Model file for the job. Use its own axes, mm. A direction names the side the tool comes from. Give positions to 0.01 mm unless a question says otherwise; leave off trailing zeros. Write each loop counter-clockwise with the first axis right and the second up, starting at its lowest first coordinate (ties: lowest second). Pieces come first, ordered by that corner, then holes. Notation, with made-up numbers: (-23, 36) - (7, 36) arc R16 ccw to (7, 52) - close; hole circle Ø2 at (-9, 88.5). An arc over 180 degrees is marked (long way). Use CSV: the item, a comma, the result in double quotes.
from build123d import *

# Parameters (mm, degrees)
BOSS_EXTRUDE1_DEPTH         = 1.524
KES_EKSTR_ZYON1_DEPTH       = 2.54
RADYUS1_R                   = 0.508
Y_KSEKLIK_EKSTR_ZYON1_DEPTH = 6.223
Y_KSEKLIK_EKSTR_ZYON2_START = -1.524
Y_KSEKLIK_EKSTR_ZYON2_DEPTH = 1.524
IZIM5_W                     = 1.905
IZIM5_H                     = 23.876
KES_EKSTR_ZYON2_DEPTH       = 9.779
RADYUS2_R                   = 0.254


with BuildPart() as part:
    # Sketch2 → Boss-Extrude1 (new body)
    with BuildSketch(Plane(origin=(0, 0, 0), x_dir=(0, 0, -1), z_dir=(1, 0, 0))):
        with BuildLine():
            Line((-10.16, 10.851579944), (-10.16, 9.756379827))
            ThreePointArc((-10.16, 9.756379827), (-8.902698353, 7.16361824), (-6.088278228, 6.54534691))
            ThreePointArc((-6.088278228, 6.54534691), (-1.097578785, 7.201770952), (3.920718614, 6.808496661))
            ThreePointArc((3.920718614, 6.808496661), (7.044965017, 7.926917254), (7.619757818, 11.195157369))
            ThreePointArc((7.619757818, 11.195157369), (4.593793799, 26.843864795), (6.687175028, 42.644379261))
            ThreePointArc((6.687175028, 42.644379261), (5.465660141, 45.611386582), (2.312998216, 45.014767901))
            ThreePointArc((2.312998216, 45.014767901), (-6.944233805, 29.036045126), (-10.16, 10.851579944))
        make_face()
    extrude(amount=BOSS_EXTRUDE1_DEPTH)

    # Sketch3 → Kes-Ekstrüzyon1 (cut)
    with BuildSketch(Plane(origin=(1.524, 0, 0), x_dir=(0, 0, -1), z_dir=(1, 0, 0))):
        with BuildLine():
            Line((-7.62, 10.851579944), (-7.62, 9.756379827))
            ThreePointArc((-7.62, 9.756379827), (-7.329853466, 9.15805023), (-6.680371899, 9.015372231))
            ThreePointArc((-6.680371899, 9.015372231), (-1.164335672, 9.74089354), (4.382203558, 9.306221955))
            ThreePointArc((4.382203558, 9.306221955), (5.103183497, 9.564319015), (5.23582799, 10.318528273))
            ThreePointArc((5.23582799, 10.318528273), (2.05490982, 26.768577734), (4.25548932, 43.378207999))
            ThreePointArc((4.25548932, 43.378207999), (-4.558282485, 28.164933022), (-7.62, 10.851579944))
        make_face()
    extrude(amount=-KES_EKSTR_ZYON1_DEPTH, mode=Mode.SUBTRACT)

    # Radyus1
    radyus1_edges = [part.edges().sort_by_distance(p)[0] for p in [
        (0.762, 43.378207999, -4.25548932),
    ]]
    fillet(radyus1_edges, radius=RADYUS1_R)

    # Çizim3 → Yükseklik-Ekstrüzyon1 (add)
    with BuildSketch(Plane.ZY):
        with BuildLine():
            Line((8.89, 9.756379827), (8.89, 10.851579944))
            ThreePointArc((8.89, 10.851579944), (6.172491894, 27.401227257), (-1.694641367, 42.212840631))
            ThreePointArc((-1.694641367, 42.212840631), (-3.87996363, 42.737551733), (-4.833471032, 40.702415677))
            ThreePointArc((-4.833471032, 40.702415677), (-3.373946338, 25.609481831), (-6.427792904, 10.756842821))
            ThreePointArc((-6.427792904, 10.756842821), (-6.074074257, 8.745618135), (-4.151461086, 8.057359308))
            ThreePointArc((-4.151461086, 8.057359308), (1.130957229, 8.471332246), (6.384325063, 7.78035957))
            ThreePointArc((6.384325063, 7.78035957), (8.116275909, 8.160834235), (8.89, 9.756379827))
        make_face()
        with BuildLine():
            Line((7.62, 10.851579944), (7.62, 9.756379827))
            ThreePointArc((7.62, 9.756379827), (7.329853466, 9.15805023), (6.680371899, 9.015372231))
            ThreePointArc((6.680371899, 9.015372231), (1.164335672, 9.74089354), (-4.382203558, 9.306221955))
            ThreePointArc((-4.382203558, 9.306221955), (-5.103183497, 9.564319015), (-5.23582799, 10.318528273))
            ThreePointArc((-5.23582799, 10.318528273), (-2.10574247, 25.541961828), (-3.601704042, 41.011689155))
            ThreePointArc((-3.601704042, 41.011689155), (-3.329273356, 41.593156599), (-2.704895567, 41.443239142))
            ThreePointArc((-2.704895567, 41.443239142), (4.96917921, 26.995100943), (7.62, 10.851579944))
        make_face(mode=Mode.SUBTRACT)
    extrude(amount=Y_KSEKLIK_EKSTR_ZYON1_DEPTH)

    # Sketch5 → Yükseklik-Ekstrüzyon2 (add)
    with BuildSketch(Plane(origin=(1.524, 0, 0), x_dir=(0, 0, -1), z_dir=(1, 0, 0)).offset(Y_KSEKLIK_EKSTR_ZYON2_START)):
        with BuildLine():
            Line((7.009110806, 43.67080126), (6.148171078, 49.106560771))
            ThreePointArc((6.148171078, 49.106560771), (3.588810081, 46.474083877), (1.217761815, 43.67080126))
            Line((1.217761815, 43.67080126), (6.534669415, 42.12894069))
            ThreePointArc((6.534669415, 42.12894069), (6.765621389, 42.901799905), (7.009110806, 43.67080126))
        make_face()
    extrude(amount=Y_KSEKLIK_EKSTR_ZYON2_DEPTH)

    # Çizim5 → Kes-Ekstrüzyon2 (cut)
    with BuildSketch(Plane.XY):
        with Locations((-5.2705, 25.4)):
            Rectangle(IZIM5_W, IZIM5_H)
    extrude(amount=-KES_EKSTR_ZYON2_DEPTH, mode=Mode.SUBTRACT)

    # Radyus2
    radyus2_edges = [part.edges().sort_by_distance(p)[0] for p in [
        (1.524, 31.644607634, 5.912857567),
        (1.524, 10.303979886, 10.16),
        (1.524, 7.16361824, 8.902698353),
        (1.524, 7.201770952, 1.097578785),
        (1.524, 7.926917254, -7.044965017),
        (1.524, 9.74089354, 1.164335672),
        (1.524, 10.303979886, 7.62),
        (1.524, 9.15805023, 7.329853466),
        (1.524, 9.564319015, -5.103183497),
        (1.524, 27.381577524, -4.580766254),
        (1.524, 26.995100943, 4.96917921),
        (1.524, 25.541961828, -2.10574247),
        (1.524, 41.593156599, -3.329273357),
        (1.524, 46.388681016, -6.578640942),
    ]]
    fillet(radyus2_edges, radius=RADYUS2_R)


solid = part.part
(1) Flat gauge pins, fed straight in: P1, Ø4, axis at x = 0, y = 27, coming from the +Z side; P2, Ø5, axis at y = 27.5, z = -4, coming from the -X side; P3, Ø1.5, axis at x = -4.5, y = 23.5, coming from the -Z side. Where does each tip first touch, or does it go through?
Checked values:
P1,"stops at z = 8.24"
P2,"stops at x = -4.32"
P3,"stops at z = -3.6"
(2) Wall check: probe 1 along Z at (x, y) = (-2.5, 10); probe 2 along Z at (x, y) = (-1, 18); probe 3 along Y at (x, z) = (-4.5, 3.25). Give the ranges that are in metal, low to high. Write a range as [from, to].
Checked values:
probe 1,"z = [-6.55, -5.28], [7.62, 8.89]"
probe 2,"z = [-4.36, -3.06], [7.11, 8.39]"
probe 3,"y = [8.33, 9.6], [31.4, 34.35]"
(3) Saw through at A-A, the plane x = -3.75. List the corners of the cut face in (y, z) (1 decimal).
Checked values:
outline,"(7.8, 6.4) arc R25.4 cw to (8.1, -4.2) arc R2 ccw to (10.8, -6.4) arc R50.9 cw to (40.7, -4.8) arc R1.8 ccw to (42.2, -1.7) arc R51.8 ccw to (10.9, 8.9) - (9.8, 8.9) arc R2 ccw to start; hole (9, 6.7) arc R26.7 cw to (9.3, -4.4) arc R0.8 ccw to (10.3, -5.2) arc R52.1 cw to (41, -3.6) arc R0.5 ccw to (41.4, -2.7) arc R50.5 ccw to (10.9, 7.6) - (9.8, 7.6) arc R0.8 ccw to start"
(4) 3-axis set-ups, long thin cutter, end or side, ignore diameter. For faces 1 (the face through (-5, 37.338, -3)), 2 (the face through (-3, 10, 8.89)), 3 (the face through (-3.068, 8.473, 1.057)), 4 (the face through (-2.424, 9.164, 7.337)), 5 (the face through (-3.068, 27.178, 6.247)): which of +Z, -Z, +X, -X, +Y, -Y reach the whole face in a straight line?
Checked values:
face 1,"-Z, -X"
face 2,"+Z, -X, +Y, -Y"
face 3,"-X, -Y"
face 4,"+X, -X"
face 5,"+Z, -X, +Y"
